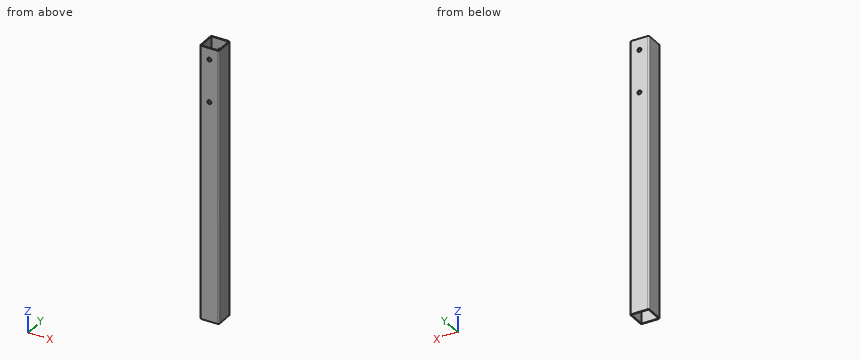
Autodesk Inventor part; units mm, degrees
ref_plane "YZ Plane" through (0, 0, 0) normal (1, 0, 0) x (0, 1, 0)
ref_plane "XZ Plane" through (0, 0, 0) normal (0, 1, 0) x (-1, 0, 0)
ref_plane "XY Plane" through (0, 0, 0) normal (0, 0, 1) x (1, 0, 0)
sketch "Sketch1" plane through (0, 0, 0) normal (0, 0, 1) x (1, 0, 0)
  line L0 (7.9375, -7.9375) -> (-7.9375, -7.9375)
  line L1 (-7.9375, -7.9375) -> (-7.9375, 7.9375)
  line L2 (-7.9375, 7.9375) -> (7.9375, 7.9375)
  line L3 (7.9375, 7.9375) -> (7.9375, -7.9375)
  line L4 (-7.1437, -7.1438) -> (-7.1437, 7.1437)
  line L5 (-7.1437, 7.1437) -> (7.1437, 7.1438)
  line L6 (7.1437, 7.1438) -> (7.1438, -7.1437)
  line L7 (7.1438, -7.1437) -> (-7.1437, -7.1438)
  line L8 (0, 0) -> (5.5522, 0)
  point P0 (0, 0)
  point P1 (0, 0)
  point P2 (0, 0)
  dimension "d4" = 45
  dimension "d5" = 14.2875
  dimension "d6" = 15.875
extrude "Extrusion1" add sketch "Sketch1" along normal blind 228.6
sketch "Sketch2" plane through (-7.9375, 7.9375, 0) normal (0, 1, 0) x (1, 0, 0)
  line L0 (0, -228.6) -> (15.875, -228.6)
  line L1 (15.875, 0) -> (15.875, -228.6)
  line L2 (0, 0) -> (0, -228.6)
  line L3 (7.9375, -228.6) -> (7.9375, -257.0929)
  line L4 (7.9375, -219.075) -> (26.9875, -219.075) construction
  point P0 (7.9375, 0)
  point P1 (7.9375, -183.515)
  dimension "d27" = 9.525
  dimension "d30" = 35.56
hole "Hole1" at (0, 7.9375, 219.075) at (0, 7.9375, 183.515) direction (0, -1, 0) diameter 3.302 end through all
fillet "Fillet1" radius 1.27 4 edges at (-7.9375, 7.9375, 114.3) (7.9375, 7.9375, 114.3) (7.9375, -7.9375, 114.3) (-7.9375, -7.9375, 114.3)
properties part number "Arm"
Could you check a few things on this model? Use its own coordinates, in mm. Give positions to 0.01 mm unless a question says otherwise; leave off trailing zeros. Write each loop counter-clockwise with the first axis right and the second up, starting at its lowest first coordinate (ties: lowest second). Pieces come first, ordered by that corner, then holes. Notation, with made-up numbers: (-21, -2) -> (22, -2) arc R15 cw to (22, 4) -> close; hole circle Ø6 at (53, 56). An arc over 180 degrees is marked (long way). Answer as a JSON object with one key per item and string values.
Q1. Suppose I cut it at A-A on z = 208. Write out the boundary of the cut face in (x, y), then the cut area to 3 significant figures.
Taken from the geometry:
{"outline": "(-7.94, -6.67) arc R1.27 ccw to (-6.67, -7.94) -> (6.67, -7.94) arc R1.27 ccw to (7.94, -6.67) -> (7.94, 6.67) arc R1.27 ccw to (6.67, 7.94) -> (-6.67, 7.94) arc R1.27 ccw to (-7.94, 6.67) -> close; hole (-7.14, -7.14) -> (7.14, -7.14) -> (7.14, 7.14) -> (-7.14, 7.14) -> close", "area": "46.5 mm²"}
Q2. Suppose I cut it at B-B on y = -2.75. Write out the boundary of the cut face in (x, z).
Taken from the geometry:
{"outline": "(-7.94, 0) -> (-7.14, 0) -> (-7.14, 228.6) -> (-7.94, 228.6) -> close; (7.14, 0) -> (7.94, 0) -> (7.94, 228.6) -> (7.14, 228.6) -> close"}
Q3. Will these pins go through, and if not, where does the flat tip stop? pin 1 Ø2.5 at (x, z) = (0, 219.075) entering from -Y; pin 2 Ø5.5 at (x, z) = (0, 183.515) entering from -Y.
Taken from the geometry:
{"pin 1": "passes through", "pin 2": "stops at y = -7.94"}
Q4. Please list where this line runs through material, in increasing order: L1, parallel to X at y = -3, z = 196.
Taken from the geometry:
{"L1": "x = -7.94 to -7.14, 7.14 to 7.94"}
